Design review of the part built by this model. Coordinates are the model's own, in mm. A direction names the side the tool comes from. Give positions to 0.01 mm unless a question says otherwise; leave off trailing zeros. Loops run counter-clockwise (first coordinate to the right, second up) from the corner with the lowest first, then second, coordinate; pieces in that order, holes last. Notation, with made-up numbers: (67, 30) - (108, 30) arc R27 cw to (108, 66) - close; hole circle Ø7 at (-32.75, 14.25). An arc over 180 degrees is marked (long way). Write each question's results on one line, items separated by ' | '.
```python
from build123d import *

# Parameters (mm, degrees)
SKETCH_W     = 51
SKETCH_H     = 20
PAD_DEPTH    = 2
PAD001_DEPTH = 12


with BuildPart() as part:
    # Sketch → Pad (new body)
    with BuildSketch(Plane.XY):
        with Locations((25.5, 10)):
            Rectangle(SKETCH_W, SKETCH_H)
    extrude(amount=PAD_DEPTH)

    # Sketch001 (on Face6 of Pad) → Pad001 (join)
    with BuildSketch(Plane.XY.offset(2)):
        with BuildLine():
            Line((1.5, 1.5), (1.5, 17))
            ThreePointArc((3, 18.5), (1.93934, 18.06066), (1.5, 17))
            Line((3, 18.5), (48, 18.5))
            ThreePointArc((49.5, 17), (49.06066, 18.06066), (48, 18.5))
            Line((49.5, 17), (49.5, 1.5))
            Line((49.5, 1.5), (47.5, 1.5))
            Line((47.5, 1.5), (47.5, 16.5))
            Line((47.5, 16.5), (3.5, 16.5))
            Line((3.5, 16.5), (3.5, 1.5))
            Line((3.5, 1.5), (1.5, 1.5))
        make_face()
    extrude(amount=PAD001_DEPTH)


solid = part.part
```
Item 1: Tool access review of faces 1 (the face through (49.07, 18.05, 7.92)), 2 (the face through (3.5, 9, 8)), 3 (the face through (3, 1.5, 8)), 4 (the face through (1.5, 9, 8)): name each direction out of +Z, -Z, +X, -X, +Y, -Y from which nothing blocks a thin tool from reaching the whole face with its end or side.
Output values:
face 1: +Z, +X, +Y | face 2: +Z, -Y | face 3: +Z, +X, -X, -Y | face 4: +Z, -X, +Y, -Y
Item 2: Wall thickness on probe 1 along X at (y, z) = (12.75, 9); probe 2 along Z at (x, y) = (37, 1.75); probe 3 along Y at (x, z) = (4.5, 7.75): over which ranges is each line inside the solid? List them lowest first.
Output values:
probe 1: x = 1.5 to 3.5, 47.5 to 49.5 | probe 2: z = 0 to 2 | probe 3: y = 16.5 to 18.5
Item 3: We need section A-A on y = 7.75. Give the boundary of the cut face in (x, z), then the cut area to 3 significant figures.
Output values:
outline: (0, 0) - (51, 0) - (51, 2) - (49.5, 2) - (49.5, 14) - (47.5, 14) - (47.5, 2) - (3.5, 2) - (3.5, 14) - (1.5, 14) - (1.5, 2) - (0, 2) - close | area: 150 mm²
Item 4: We need section C-C on z = 8. Give the boundary of the cut face in (x, y), then the cut area to 3 significant figures.
Output values:
outline: (1.5, 1.5) - (3.5, 1.5) - (3.5, 16.5) - (47.5, 16.5) - (47.5, 1.5) - (49.5, 1.5) - (49.5, 17) arc R1.5 ccw to (48, 18.5) - (3, 18.5) arc R1.5 ccw to (1.5, 17) - close | area: 155 mm²
Item 5: We need section B-B on x = 15. Give the boundary of the cut face in (y, z), then the cut area to 3 significant figures.
Output values:
outline: (0, 0) - (20, 0) - (20, 2) - (18.5, 2) - (18.5, 14) - (16.5, 14) - (16.5, 2) - (0, 2) - close | area: 64.0 mm²
Item 6: Draft analysis for pull direction X (two halves, no side actions). For faces 5 (the face through (1.95, 18.07, 7.92)), 6 (the face through (26, 16.5, 8)), 7 (the face through (49.5, 9, 8)), state which applies: +X half, -X half, draft (parallel to the pull), parting line (faces both ways), or undercut.
Output values:
face 5: -X half | face 6: undercut | face 7: +X half
Item 7: Clearance check with flat-ended pins moving along their axes: P1, Ø3.5, axis at x = 31.5, z = 9, coming from the +Y side; P2, Ø1.5, axis at x = 33, z = 7, coming from the -Y side; P3, Ø8, axis at x = 19.5, y = 5, coming from the +Z side. State where each tip first meets the part, or that it passes through.
Output values:
P1: stops at y = 18.5 | P2: stops at y = 16.5 | P3: stops at z = 2
